The listing builds one solid part. Answer for the finished solid, in the listing's coordinates (mm). Face numbers are marked on the shaded views. Give positions to 0.01 mm unless a question says otherwise; leave off trailing zeros. Loops run counter-clockwise (first coordinate to the right, second up) from the corner with the lowest first, then second, coordinate; pieces in that order, holes last. Notation, with made-up numbers: M 72,70.25 L 97,70.25 A21 cw 97,103.25 Z; hole C 76,45.25 d11. An arc over 180 degrees is marked long. One line per item, written item: value. Start each with the question number.
Q1. A flat-ended cylindrical pin translates along its axis: pin 1 (2 mm diameter, centred on x = 3, z = 3.5, fed in from -Y). Find the tip coordinate at first contact, or state that the pin passes through.
Q2. The mould has two halves that part along Z. Classify the marked faces 1 and 2: +Z half, -Z half, draft (parallel to the pull), parting line (faces both ways), or undercut.
Q3. A cutting plane is placed at C-C, the plane x = -4. Determine the outline of the cut face in (y, z).
Q4. A cutting plane is placed at A-A, the plane x = 15. Determine the outline of the cut face in (y, z).
Q5. Consider L1, parallel to Y at x = -17, z = 1.15; L2, parallel to X at y = 20, z = 1.35; L3, parallel to Y at x = 1.5, z = 2.1. Determine where each line is inside the solid, lowest interval first.
Q6. A cutting plane is placed at D-D, the plane x = -23.5. Determine the outline of the cut face in (y, z), and give its area (3 significant figures).
Q7. A cutting plane is placed at B-B, the plane z = 1.45. Determine the outline of the cut face in (x, y) (3 decimals), and give its area (3 significant figures).
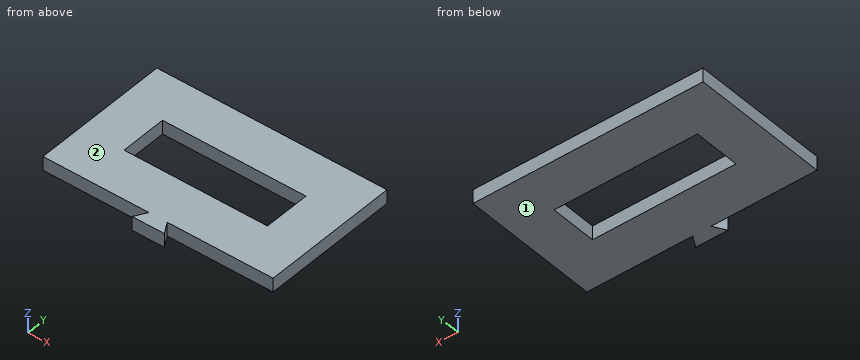
from build123d import *

# Parameters (mm, degrees)
F1_DEPTH = 3.81


with BuildPart() as f1:
    # F0 (on Top) → F1 (new body)
    with BuildSketch(Plane.XY):
        Polygon((-34.29, 0), (-5.08, 0), (-6.985, -3.299557), (1.905, -3.299557), (0, 0), (29.21, 0), (29.21, 38.1), (-2.54, 38.1), (-34.29, 38.1), align=None)
        Polygon((-22.3266, 25.4762), (-2.54, 25.4762), (17.2466, 25.4762), (17.2466, 12.6238), (-22.3266, 12.6238), align=None, mode=Mode.SUBTRACT)
    extrude(amount=F1_DEPTH)


solid = f1.part
Answer block:
1. pin 1: y = 0
2. face 1: -Z half
2. face 2: +Z half
3. outline: M -3.3,0 L 12.62,0 L 12.62,3.81 L -3.3,3.81 Z; M 25.48,0 L 38.1,0 L 38.1,3.81 L 25.48,3.81 Z
4. outline: M 0,0 L 12.62,0 L 12.62,3.81 L 0,3.81 Z; M 25.48,0 L 38.1,0 L 38.1,3.81 L 25.48,3.81 Z
5. L1: 0 to 12.62, 25.48 to 38.1
5. L2: -34.29 to -22.33, 17.25 to 29.21
5. L3: -3.3 to -2.6, 0 to 12.62, 25.48 to 38.1
6. outline: M 0,0 L 38.1,0 L 38.1,3.81 L 0,3.81 Z
6. area: 145 mm^2
7. outline: M -34.29,0 L -5.08,0 L -6.985,-3.3 L 1.905,-3.3 L 0,0 L 29.21,0 L 29.21,38.1 L -34.29,38.1 Z; hole M -22.327,12.624 L 17.247,12.624 L 17.247,25.476 L -22.327,25.476 Z
7. area: 1,930 mm^2
